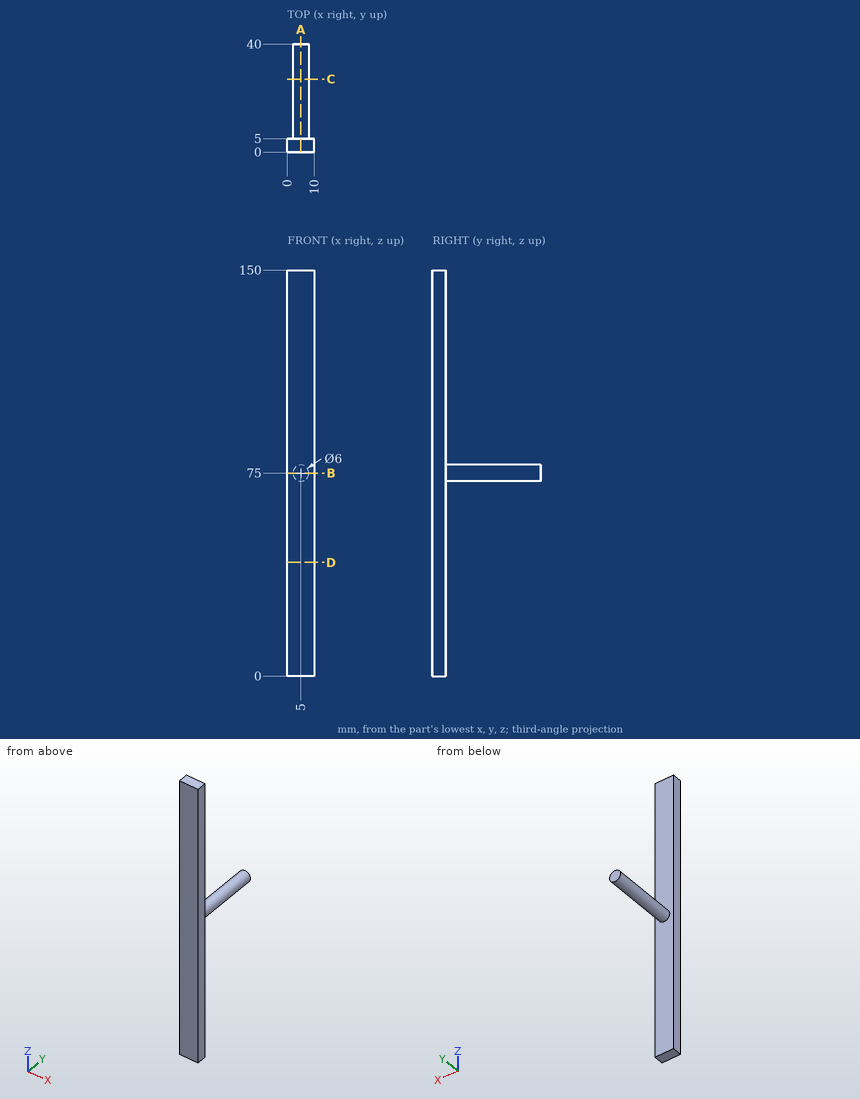
Here's the drawing with two shaded views (mm, measured from the low corner). I have some questions. Coordinates: 2 decimals unless noted, no trailing zeros. Order: outer loops, then holes, each group sorted by start corner. A loop starts at its lowest first (then second) coordinate and runs counter-clockwise, first axis right, second up.
Item 1: If we section it at A-A on x = 5: List the corners of the cut face in (y, z) for me.
Result sheet:
outline: (0, 0) - (5, 0) - (5, 72) - (40, 72) - (40, 78) - (5, 78) - (5, 150) - (0, 150) - close
Item 2: For P1, Ø1.5, axis at x = 6, z = 38.5, coming from the -Y side; P2, Ø3, axis at x = 3.5, z = 44, coming from the +Y side; P3, Ø3, axis at x = 7, y = 12.5, coming from the +Z side; P4, Ø6, axis at x = 1, y = 19, coming from the -Z side, each with a flat end and sliding along its axis, tell me the tip position at first contact or that it passes through.
Result sheet:
P1: stops at y = 0
P2: stops at y = 5
P3: stops at z = 77.96
P4: stops at z = 72.17
Item 3: If we section it at B-B on z = 75: List the corners of the cut face in (x, y) for me, plus the area to 3 significant figures.
Result sheet:
outline: (0, 0) - (10, 0) - (10, 5) - (8, 5) - (8, 40) - (2, 40) - (2, 5) - (0, 5) - close
area: 260 mm2
Item 4: I need wall thicknesses on line 1 (Y direction, x = 1.5, z = 16); line 2 (Z direction, x = 5.75, y = 5.5); line 3 (Z direction, x = 7.5, y = 27.5). Which ranges of each line are inside material? Lowest first, please.
Result sheet:
line 1: y = 0 to 5
line 2: z = 72.1 to 77.9
line 3: z = 73.34 to 76.66
Item 5: If we section it at C-C on y = 27: List the corners of the cut face in (x, z) for me.
Result sheet:
outline: circle Ø6 at (5, 75)
Item 6: If we section it at D-D on z = 42: List the corners of the cut face in (x, y) for me, plus the area to 3 significant figures.
Result sheet:
outline: (0, 0) - (10, 0) - (10, 5) - (0, 5) - close
area: 50.0 mm2
